from build123d import *

# Parameters (mm, degrees)
SKETCH1_R           = 3.65
SKETCH1_R_2         = 2.4
SKETCH1_R_3         = 1.6
SKETCH1_R_4         = 0.5
BOSS_EXTRUDE1_DEPTH = 1.6
SKETCH1_3_R         = 3.65
SKETCH1_3_R_2       = 2.4
BOSS_EXTRUDE2_DEPTH = 6
SKETCH1_4_R         = 2.4
SKETCH1_4_R_2       = 1.6
CUT_EXTRUDE1_DEPTH  = 1


with BuildPart() as part:
    # Sketch1 → Boss-Extrude1 (new body)
    # profile 1 of 3: a face of its own
    with BuildSketch(Plane(origin=(0, 0, 0), x_dir=(1, 0, 0), z_dir=(0, 1, 0))):
        with Locations((-17.661574497, 0)):
            Circle(SKETCH1_R)
        with Locations((-17.661574497, 0)):
            Circle(SKETCH1_R_2, mode=Mode.SUBTRACT)
    # profile 2 of 3: a face of its own
    with BuildSketch(Plane(origin=(0, 0, 0), x_dir=(1, 0, 0), z_dir=(0, 1, 0))):
        with Locations((-17.661574497, 0)):
            Circle(SKETCH1_R_2)
        with Locations(Location((-17.661574497, 0, 0), (0, 0, 270))):
            Circle(SKETCH1_R_3, mode=Mode.SUBTRACT)
    # profile 3 of 3: a face of its own
    with BuildSketch(Plane(origin=(0, 0, 0), x_dir=(1, 0, 0), z_dir=(0, 1, 0))):
        with BuildLine():
            Line((-4.119202068, 1.95), (-15.320100602, 2.8))
            ThreePointArc((-15.320100602, 2.8), (-14.35484804, 1.545334961), (-14.011574497, 0))
            ThreePointArc((-14.011574497, 0), (-14.35484804, -1.545334961), (-15.320100602, -2.8))
            Line((-15.320100602, -2.8), (-4.119202068, -1.95))
            ThreePointArc((-4.119202068, -1.95), (-2.311574497, 0), (-4.119202068, 1.95))
        make_face()
        with Locations(Location((-13.331400804, 0, 0), (0, 0, 270))):
            Circle(SKETCH1_R_4, mode=Mode.SUBTRACT)
        with Locations(Location((-11.331400804, 0, 0), (0, 0, 270))):
            Circle(SKETCH1_R_4, mode=Mode.SUBTRACT)
        with Locations(Location((-9.331400804, 0, 0), (0, 0, 270))):
            Circle(SKETCH1_R_4, mode=Mode.SUBTRACT)
        with Locations(Location((-7.331400804, 0, 0), (0, 0, 270))):
            Circle(SKETCH1_R_4, mode=Mode.SUBTRACT)
        with Locations(Location((-5.331400804, 0, 0), (0, 0, 270))):
            Circle(SKETCH1_R_4, mode=Mode.SUBTRACT)
        with Locations(Location((-3.331400804, 0, 0), (0, 0, 270))):
            Circle(SKETCH1_R_4, mode=Mode.SUBTRACT)
    extrude(amount=BOSS_EXTRUDE1_DEPTH)

    # Sketch1<3> → Boss-Extrude2 (add)
    with BuildSketch(Plane(origin=(0, 0, 0), x_dir=(1, 0, 0), z_dir=(0, 1, 0))):
        with Locations(Location((-17.661574497, 0, 0), (0, 0, 50.096260743))):
            Circle(SKETCH1_3_R)
        with Locations(Location((-17.661574497, 0, 0), (0, 0, 270))):
            Circle(SKETCH1_3_R_2, mode=Mode.SUBTRACT)
    extrude(amount=BOSS_EXTRUDE2_DEPTH)

    # Sketch1<4> → Cut-Extrude1 (cut)
    with BuildSketch(Plane(origin=(0, 0, 0), x_dir=(1, 0, 0), z_dir=(0, 1, 0))):
        with Locations(Location((-17.661574497, 0, 0), (0, 0, 270))):
            Circle(SKETCH1_4_R)
        with Locations(Location((-17.661574497, 0, 0), (0, 0, 270))):
            Circle(SKETCH1_4_R_2, mode=Mode.SUBTRACT)
    extrude(amount=CUT_EXTRUDE1_DEPTH, mode=Mode.SUBTRACT)


solid = part.part
For this review, take the finished solid that the model builds, in its own axes (mm). A direction names the side the tool comes from. Round coordinates to 2 decimals unless told otherwise and drop trailing zeros. Order: outer loops, then holes, each group sorted by start corner. A loop starts at its lowest first (then second) coordinate and runs counter-clockwise, first axis right, second up. Notation, with made-up numbers: M 43,22 L 71,22 A20 ccw 71,44 Z; hole C 64,37.5 d7. An arc over 180 degrees is marked long. Use a Markdown table: item, result. Add a question column.
Item 1: Add section A-A, the plane z = 0. State how many separate pieces and enclosed holes the cut face has, then the cut area to 3 significant figures.
Item 2: Tool access review of faces 4 (the flat face through (-15, 6, 1)), 5 (the cylindrical face through (-20.005, 3.769, -0.52)), 6 (the flat face through (-18, 1, 2)): name each direction out of +Z, -Z, +X, -X, +Y, -Y from which nothing blocks a thin tool from reaching the whole face with its end or side.
Item 3: To check wall thickness, follow line 1 along X through (y, z) = (2.7, 0); line 2 along Y through (x, z) = (-9, 1.75); line 3 along Y through (x, z) = (-19.5, -1.5). State the ranges of each line that lie inside material, in increasing order.
Item 4: Insertion check: pin 1 (4 mm diameter, centred on x = -7, z = -2.5, fed in from +Y); pin 2 (3 mm diameter, centred on y = 4, z = -1.5, fed in from +X). Each pin has a flat end and moves straight along its axis. Give the tip position at first contact, or say it passes through.
Item 5: Add section C-C, the plane z = 0.75. Give the boundary of the cut face in (x, y), then the cut area to 3 significant figures.
Item 6: Mouldability with a two-part tool opening along X and no side actions: class faces 1 (the flat face through (-9.64, 0.79, -2.37)), 2 (the cylindrical face through (-21.28, 2.96, 0.48)), 3 (the flat face through (-17, 1.6, 2)) as released by +X, released by -X, zero draft, split by the parting line, or undercut.
Item 7: Add section D-D, the plane y = 3.45. Give the boundary of the cut face in (x, z).
Item 8: Add section B-B, the plane x = -18.5. Give the boundary of the cut face in (y, z), then the cut area to 3 significant figures.
Geometry results:
| question | item | result |
|---|---|---|
| 1 | separate pieces | 8 |
| 1 | enclosed holes | 0 |
| 1 | area | 25.1 mm² |
| 2 | face 4 | +Z, -Z, +X, -X, +Y |
| 2 | face 5 | +Y |
| 2 | face 6 | -Y |
| 3 | line 1 | x = -21.31 to -20.06, -15.26 to -14.01 |
| 3 | line 2 | y = 0 to 1.6 |
| 3 | line 3 | y = 1 to 1.6 |
| 4 | pin 1 | stops at y = 1.6 |
| 4 | pin 2 | stops at x = -14.01 |
| 5 | outline | M -21.23,0 L -19.94,0 L -19.94,1 L -19.07,1 L -19.07,1.6 L -19.94,1.6 L -19.94,6 L -21.23,6 Z; M -16.25,1 L -15.38,1 L -15.38,0 L -2.46,0 L -2.46,1.6 L -14.09,1.6 L -14.09,6 L -15.38,6 L -15.38,1.6 L -16.25,1.6 Z |
| 5 | area | 35.2 mm² |
| 6 | face 1 | released by +X |
| 6 | face 2 | split by the parting line |
| 6 | face 3 | undercut |
| 7 | outline | C -17.66,0 d7.3; hole C -17.66,0 d4.8 |
| 8 | outline | M 0,-3.55 L 6,-3.55 L 6,-2.25 L 1.6,-2.25 L 1.6,-1.36 L 1,-1.36 L 1,-2.25 L 0,-2.25 Z; M 0,2.25 L 1,2.25 L 1,1.36 L 1.6,1.36 L 1.6,2.25 L 6,2.25 L 6,3.55 L 0,3.55 Z |
| 8 | area | 16.7 mm² |
